from build123d import *

# Parameters (mm, degrees)
SKETCH1_R           = 8
BOSS_EXTRUDE1_DEPTH = 7
SKETCH2_R           = 6
BOSS_EXTRUDE2_DEPTH = 8
SKETCH3_R           = 8
BOSS_EXTRUDE3_DEPTH = 1
CUT_EXTRUDE1_REACH  = 21.596
SKETCH4_R           = 2.25


with BuildPart() as part:
    # Sketch1 → Boss-Extrude1 (new body)
    with BuildSketch(Plane(origin=(0, 0, 0), x_dir=(1, 0, 0), z_dir=(0, 1, 0))):
        with Locations(Location((0, 0, 0), (0, 0, 270))):
            Circle(SKETCH1_R)
    extrude(amount=BOSS_EXTRUDE1_DEPTH)

    # Sketch2 → Boss-Extrude2 (add)
    with BuildSketch(Plane(origin=(0, 7, 0), x_dir=(1, 0, 0), z_dir=(0, 1, 0))):
        with Locations(Location((0, 0, 0), (0, 0, 270))):
            Circle(SKETCH2_R)
    extrude(amount=BOSS_EXTRUDE2_DEPTH)

    # Sketch3 → Boss-Extrude3 (add)
    with BuildSketch(Plane(origin=(0, 15, 0), x_dir=(1, 0, 0), z_dir=(0, 1, 0))):
        with Locations(Location((0, 0, 0), (0, 0, 270))):
            Circle(SKETCH3_R)
    extrude(amount=BOSS_EXTRUDE3_DEPTH)

    # Sketch4 → Cut-Extrude1 (cut, up to next)
    with BuildSketch(Plane(origin=(0, 16, 0), x_dir=(1, 0, 0), z_dir=(0, 1, 0)), mode=Mode.PRIVATE) as cut_extrude1_sk1:
        with Locations(Location((0, 0, 0), (0, 0, 270))):
            Circle(SKETCH4_R)
    cut_extrude1_tool1 = extrude(cut_extrude1_sk1.sketch, amount=-CUT_EXTRUDE1_REACH, mode=Mode.PRIVATE) & part.part
    add(cut_extrude1_tool1.solids().sort_by_distance((0, 16, 0))[0], mode=Mode.SUBTRACT)


solid = part.part
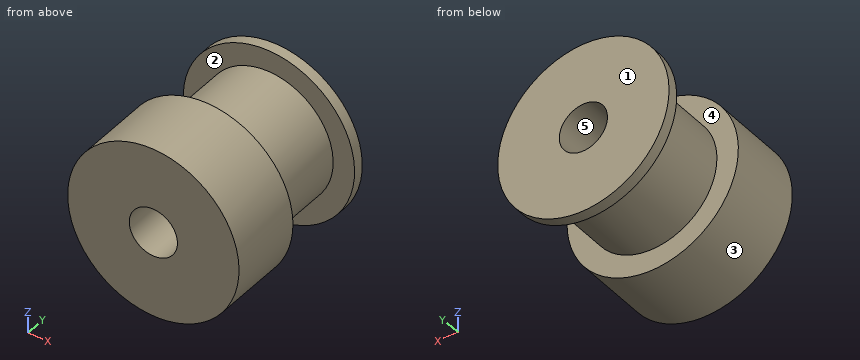
Design review of the part built by this model. Coordinates are the model's own, in mm. Face numbers are marked on the shaded views. A direction names the side the tool comes from. Coordinates: 2 decimals unless noted, no trailing zeros. Order: outer loops, then holes, each group sorted by start corner. A loop starts at its lowest first (then second) coordinate and runs counter-clockwise, first axis right, second up. Notation, with made-up numbers: M 45.5,77 L 69.5,77 A17 ccw 69.5,106 Z; hole C 86.25,-16 d4. An arc over 180 degrees is marked long. Use a Markdown table: item, result.
(1) For the marked faces 1 and 2, list the 3-axis set-ups (+Z, -Z, +X, -X, +Y, -Y) from which the entire face can be reached by the end or side of a thin tool; tool diameter is ignored.
Worked answers:
| item | result |
|---|---|
| face 1 | +Z, -Z, +X, -X, +Y |
| face 2 | none |
(2) Add section A-A (x = 0). Give the boundary of the cut face in (y, z).
Worked answers:
| item | result |
|---|---|
| outline | M 0,-8 L 7,-8 L 7,-6 L 15,-6 L 15,-8 L 16,-8 L 16,-2.25 L 0,-2.25 Z; M 0,2.25 L 16,2.25 L 16,8 L 15,8 L 15,6 L 7,6 L 7,8 L 0,8 Z |
(3) Add section B-B (z = 0). Give the boundary of the cut face in (x, y), then the cut area to 3 significant figures.
Worked answers:
| item | result |
|---|---|
| outline | M -8,0 L -2.25,0 L -2.25,16 L -8,16 L -8,15 L -6,15 L -6,7 L -8,7 Z; M 2.25,0 L 8,0 L 8,7 L 6,7 L 6,15 L 8,15 L 8,16 L 2.25,16 Z |
| area | 152 mm2 |
(4) Add section C-C (y = 9). Give the boundary of the cut face in (x, z), then the cut area to 3 significant figures.
Worked answers:
| item | result |
|---|---|
| outline | C 0,0 d12; hole C 0,0 d4.5 |
| area | 97.2 mm2 |
(5) Add section D-D (z = 5). Give the boundary of the cut face in (x, y) (3 decimals).
Worked answers:
| item | result |
|---|---|
| outline | M -6.245,0 L 6.245,0 L 6.245,7 L 3.317,7 L 3.317,15 L 6.245,15 L 6.245,16 L -6.245,16 L -6.245,15 L -3.317,15 L -3.317,7 L -6.245,7 Z |
(6) Draft analysis for pull direction Z (two halves, no side actions). For the marked faces 3, 4 and 5, state which applies: released by +Z, released by -Z, zero draft, split by the parting line, or undercut.
Worked answers:
| item | result |
|---|---|
| face 3 | split by the parting line |
| face 4 | zero draft |
| face 5 | undercut |
(7) For P1, Ø1.5, axis at y = 6, z = 1.5, coming from the +X side; P2, Ø4, axis at x = 2.5, y = 2.5, coming from the +Z side; P3, Ø6, axis at x = 5.5, y = 5, coming from the -Z side; P4, Ø6, axis at x = 0, z = 0, coming from the -Y side, all flat-tipped, find the tip position at first contact; note any pin that passes through.
Worked answers:
| item | result |
|---|---|
| P1 | stops at x = 7.96 |
| P2 | stops at z = 7.98 |
| P3 | stops at z = -7.6 |
| P4 | stops at y = 0 |
(8) Wall thickness on probe 1 along X at (y, z) = (4.75, 0); probe 2 along Y at (x, z) = (7, -1); probe 3 along X at (y, z) = (9, 0): over which ranges is each line inside the solid? List them lowest first.
Worked answers:
| item | result |
|---|---|
| probe 1 | x = -8 to -2.25, 2.25 to 8 |
| probe 2 | y = 0 to 7, 15 to 16 |
| probe 3 | x = -6 to -2.25, 2.25 to 6 |
